The model under review builds one solid part; all positions refer to its coordinate system, in mm. Face numbers are marked on the shaded views. Give positions to 0.01 mm unless a question says otherwise; leave off trailing zeros. Order: outer loops, then holes, each group sorted by start corner. A loop starts at its lowest first (then second) coordinate and runs counter-clockwise, first axis right, second up. Notation, with made-up numbers: (-13, 13.25) - (4, 13.25) arc R21 cw to (4, 38.25) - close; hole circle Ø3 at (52.25, -33). An arc over 180 degrees is marked (long way). Answer as CSV lines item,"result". Start each with the question number.
from build123d import *

# Parameters (mm, degrees)
SKETCH1_R           = 3
BOSS_EXTRUDE1_DEPTH = 3
FILLET3_R           = 0.75
FILLET4_R           = 0.75


with BuildPart() as part:
    # Sketch1 → Boss-Extrude1 (new body)
    with BuildSketch(Plane.XY):
        with BuildLine():
            Line((6, 12.755292895), (-18.5, 12.755292895))
            Line((-18.5, 12.755292895), (-18.5, 3.755292895))
            Line((-18.5, 3.755292895), (-15.5, 3.755292895))
            Line((-15.5, 3.755292895), (-15.5, 4.755292895))
            ThreePointArc((-15.5, 4.755292895), (-15.3, 5.755292895), (-15.5, 6.755292895))
            Line((-15.5, 6.755292895), (-15.5, 7.755292895))
            Line((-15.5, 7.755292895), (-12.5, 7.755292895))
            Line((-12.5, 7.755292895), (-12.5, 6.755292895))
            ThreePointArc((-12.5, 6.755292895), (-12.7, 5.755292895), (-12.5, 4.755292895))
            Line((-12.5, 4.755292895), (-12.5, -6.244707105))
            Line((-12.5, -6.244707105), (-18.5, -6.244707105))
            Line((-18.5, -6.244707105), (-18.5, -16.244707105))
            Line((-18.5, -16.244707105), (-15.5, -16.244707105))
            Line((-15.5, -16.244707105), (-15.5, -14.744707105))
            ThreePointArc((-15.5, -14.744707105), (-15.3, -13.744707105), (-15.5, -12.744707105))
            Line((-15.5, -12.744707105), (-15.5, -11.244707105))
            Line((-15.5, -11.244707105), (-12.5, -11.244707105))
            Line((-12.5, -11.244707105), (-12.5, -12.744707105))
            ThreePointArc((-12.5, -12.744707105), (-12.7, -13.744707105), (-12.5, -14.744707105))
            Line((-12.5, -14.744707105), (-12.5, -39.244707105))
            Line((-12.5, -39.244707105), (0, -39.244707105))
            Line((0, -39.244707105), (0, -14.744707105))
            ThreePointArc((0, -14.744707105), (0.2, -13.744707105), (0, -12.744707105))
            Line((0, -12.744707105), (0, -11.244707105))
            Line((0, -11.244707105), (3, -11.244707105))
            Line((3, -11.244707105), (3, -12.744707105))
            ThreePointArc((3, -12.744707105), (2.8, -13.744707105), (3, -14.744707105))
            Line((3, -14.744707105), (3, -16.244707105))
            Line((3, -16.244707105), (6, -16.244707105))
            Line((6, -16.244707105), (6, -6.244707105))
            Line((6, -6.244707105), (0, -6.244707105))
            Line((0, -6.244707105), (0, 4.755292895))
            ThreePointArc((0, 4.755292895), (0.2, 5.755292895), (0, 6.755292895))
            Line((0, 6.755292895), (0, 7.755292895))
            Line((0, 7.755292895), (3, 7.755292895))
            Line((3, 7.755292895), (3, 6.755292895))
            ThreePointArc((3, 6.755292895), (2.8, 5.755292895), (3, 4.755292895))
            Line((3, 4.755292895), (3, 3.755292895))
            Line((3, 3.755292895), (6, 3.755292895))
            Line((6, 3.755292895), (6, 12.755292895))
        make_face()
        with Locations((-6.25, -29.244707105)):
            Circle(SKETCH1_R, mode=Mode.SUBTRACT)
    extrude(amount=BOSS_EXTRUDE1_DEPTH)

    # Fillet3
    fillet3_edges = [part.edges().sort_by_distance(p)[0] for p in [
        (3, 3.755292895, 1.5),
    ]]
    fillet(fillet3_edges, radius=FILLET3_R)

    # Fillet4
    fillet4_edges = [part.edges().sort_by_distance(p)[0] for p in [
        (-15.5, 3.755292895, 1.5),
        (3, -16.244707105, 1.5),
        (-15.5, -16.244707105, 1.5),
    ]]
    fillet(fillet4_edges, radius=FILLET4_R)


solid = part.part
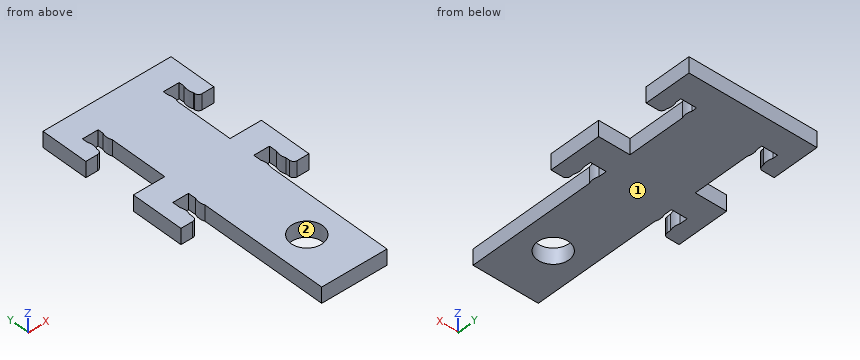
Item 1: Take a section at B-B on y = -21.5. Write out the cut boundary in (x, z), and give its area (3 significant figures).
Item 2: Take a section at A-A on x = -6.25. Write out the cut boundary in (y, z).
Item 3: Clearance check with flat-ended pins moving along their axes: pin 1 (1.5 mm diameter, centred on x = -13.5, z = 1, fed in from -Y); pin 2 (1.1 mm diameter, centred on x = 5.5, z = 1, fed in from -Y); pin 3 (1.5 mm diameter, centred on y = -1, z = 2, fed in from +X). State where each tip first meets the part, or that it passes through.
Item 4: Mouldability with a two-part tool opening along Y and no side actions: class the marked faces 1 and 2 as released by +Y, released by -Y, zero draft, split by the parting line, or undercut.
Item 5: For line 1 along X through (y, z) = (-12, 0.6); line 2 along X through (y, z) = (6, 0.75); line 3 along Y through (x, z) = (-6.25, 1), list the stretches that pass through material, from the lowest coordinate up.
Data:
1,outline,"(-12.5, 0) - (0, 0) - (0, 3) - (-12.5, 3) - close"
1,area,"37.5 mm^2"
2,outline,"(-39.24, 0) - (-32.24, 0) - (-32.24, 3) - (-39.24, 3) - close; (-26.24, 0) - (12.76, 0) - (12.76, 3) - (-26.24, 3) - close"
3,pin 1,"stops at y = -11.24"
3,pin 2,"stops at y = -16.24"
3,pin 3,"stops at x = 0"
4,face 1,"zero draft"
4,face 2,"undercut"
5,line 1,"x = -18.5 to -15.5, -12.5 to 0, 3 to 6"
5,line 2,"x = -18.5 to -15.31, -12.69 to 0.19, 2.81 to 6"
5,line 3,"y = -39.24 to -32.24, -26.24 to 12.76"
